Geometry check sheet. Reference: the model listing, model coordinates, mm. A direction names the side the tool comes from. Round coordinates to 2 decimals unless told otherwise and drop trailing zeros. Order: outer loops, then holes, each group sorted by start corner. A loop starts at its lowest first (then second) coordinate and runs counter-clockwise, first axis right, second up. Notation, with made-up numbers: (-18, 18) -> (17, 18) arc R9 cw to (17, 28) -> close; hole circle Ø4 at (19.25, 74). An arc over 180 degrees is marked (long way). Use a Markdown table: item, result. Add a question column.
Item 1: Gauge pin test, flat ends, axial feed: pin 1 Ø5 at (y, z) = (17, -25) entering from -X; pin 2 Ø5 at (x, y) = (-70, 21) entering from -Z; pin 3 Ø6 at (x, y) = (50.5, 13.5) entering from -Z; pin 4 Ø1.2 at (x, z) = (9.28, -18.77) entering from -Y. Record the tip position at first contact, or that the pin passes through.
Item 2: Material ranges on probe 1 along Z at (x, y) = (32, 7.5); probe 2 along Y at (x, z) = (-67, 5); probe 3 along X at (y, z) = (34, -22.5), recorded low to high. Write a range as [from, to].
Item 3: Sectioned sample at D-D, the plane z = 45. Record the cut outline in (x, y), and give its area (3 significant figures).
Item 4: Mould release check, pull along Y, two halves, no side actions. Record for faces 4 (the flat face through (74, 33.55, -26)), 5 (the flat face through (30, 5, 0)), 6 (the flat face through (-15.741, 5, 0)): pulls with the +Y half, pulls with the -Y half, needs draft (parallel to the pull), parting line crosses it, or undercut.
Item 5: Set-up check for faces 1 (the cylindrical face through (-83, 2, 55)), 2 (the flat face through (-74.888, 39, -1)), 3 (the flat face through (59.112, 35, -26)): record each of +Z, -Z, +X, -X, +Y, -Y from which the full face is reachable in a straight line by a thin tool's end or side.
Item 6: Sectioned sample at A-A, the plane x = -85. Record the cut outline in (y, z), and give its area (3 significant figures).
Item 7: Sectioned sample at B-B, the plane z = -36.5. Record the cut outline in (x, y).
Item 8: Sectioned sample at C-C, the plane x = 56. Record the cut outline in (y, z), and give its area (3 significant figures).
from build123d import *

# Parameters (mm, degrees)
SKETCH1_W                           = 180
SKETCH1_H                           = 120
BOSS_EXTRUDE1_DEPTH                 = 10
SKETCH2_W                           = 48.844317462
SKETCH2_H                           = 61.818589288
BOSS_EXTRUDE2_DEPTH                 = 30
SKETCH3_W                           = 27
SKETCH3_H                           = 27
CUT_EXTRUDE1_DEPTH                  = 10
CUT_EXTRUDE5_DEPTH                  = 171.851904114
TAP_DRILL_FOR_M2_5_TAP1_D           = 2.05
TAP_DRILL_FOR_M2_5_TAP1_DEPTH       = 5
TAP_DRILL_FOR_M2_5_TAP1_CSINK_D     = 2.1
TAP_DRILL_FOR_M2_5_TAP1_CSINK_ANGLE = 92
TAP_DRILL_FOR_M2_5_TAP1_TIP         = 0.615882135
CUT_EXTRUDE6_DEPTH                  = 113.249721603
BOSS_EXTRUDE3_DEPTH                 = 49
SKETCH14_W                          = 46
SKETCH14_H                          = 41
CUT_EXTRUDE8_DEPTH                  = 5
TAP_DRILL_FOR_M2_5_TAP2_D           = 2.05
TAP_DRILL_FOR_M2_5_TAP2_DEPTH       = 5
TAP_DRILL_FOR_M2_5_TAP2_CSINK_D     = 2.1
TAP_DRILL_FOR_M2_5_TAP2_CSINK_ANGLE = 92
TAP_DRILL_FOR_M2_5_TAP2_TIP         = 0.615882135
BOSS_EXTRUDE5_DEPTH                 = 115
BOSS_EXTRUDE6_DEPTH                 = 115
SKETCH29_W                          = 30
SKETCH29_H                          = 3.45
BOSS_EXTRUDE10_DEPTH                = 10
SKETCH34_R                          = 2
CUT_EXTRUDE10_DEPTH                 = 5
SKETCH25_R                          = 2
CUT_EXTRUDE11_DEPTH                 = 5
SKETCH36_W                          = 25.507224214
SKETCH36_H                          = 51.818589288
CUT_EXTRUDE12_DEPTH                 = 5
CUT_EXTRUDE14_DEPTH                 = 171.851904114


with BuildPart() as part:
    # Sketch1 → Boss-Extrude1 (new body)
    with BuildSketch(Plane(origin=(0, 0, 0), x_dir=(1, 0, 0), z_dir=(0, 1, 0))):
        Rectangle(SKETCH1_W, SKETCH1_H)
    extrude(amount=BOSS_EXTRUDE1_DEPTH)

    # Sketch2 → Boss-Extrude2 (add)
    with BuildSketch(Plane(origin=(0, 10, 0), x_dir=(1, 0, 0), z_dir=(0, 1, 0))):
        with Locations((-50.466101441, 0)):
            Rectangle(SKETCH2_W, SKETCH2_H)
    extrude(amount=BOSS_EXTRUDE2_DEPTH)

    # Sketch3 → Cut-Extrude1 (cut)
    with BuildSketch(Plane.ZY.offset(74.888260172)):
        with Locations((0, 25)):
            Rectangle(SKETCH3_W, SKETCH3_H)
    extrude(amount=-CUT_EXTRUDE1_DEPTH, mode=Mode.SUBTRACT)

    # Sketch4 → Cut-Extrude5 (cut, through all)
    with BuildSketch(Plane.ZY.offset(64.888260172)):
        with BuildLine():
            Line((-6.024531525, 38.226394973), (5.549516036, 38.226394973))
            ThreePointArc((5.549516036, 38.226394973), (6.551598076, 37.224312933), (5.549516036, 36.222230893))
            Line((5.549516036, 36.222230893), (-6.024531525, 36.222230893))
            ThreePointArc((-6.024531525, 36.222230893), (-7.026613565, 37.224312933), (-6.024531525, 38.226394973))
        make_face()
    extrude(amount=-CUT_EXTRUDE5_DEPTH, mode=Mode.SUBTRACT)

    # Tap Drill for M2.5 Tap1
    with Locations(Plane(origin=(-64.888260172, 36.953397965, -12.070360422), x_dir=(0, 0, -1), z_dir=(-1, 0, 0))):
        with Locations((0, 0), (-24.059553717, -0.049505255), (-23.988973263, 23.863567836), (-0.227588633, 23.863567836)):
            CounterSinkHole(TAP_DRILL_FOR_M2_5_TAP1_D / 2, TAP_DRILL_FOR_M2_5_TAP1_CSINK_D / 2, depth=TAP_DRILL_FOR_M2_5_TAP1_DEPTH, counter_sink_angle=TAP_DRILL_FOR_M2_5_TAP1_CSINK_ANGLE)
            with Locations((0, 0, -(TAP_DRILL_FOR_M2_5_TAP1_DEPTH + TAP_DRILL_FOR_M2_5_TAP1_TIP / 2))):  # 118° drill point
                Cone(0, TAP_DRILL_FOR_M2_5_TAP1_D / 2, TAP_DRILL_FOR_M2_5_TAP1_TIP, mode=Mode.SUBTRACT)

    # Sketch9 → Cut-Extrude6 (cut, through all)
    with BuildSketch(Plane(origin=(0, 10, 0), x_dir=(1, 0, 0), z_dir=(0, 1, 0))):
        with BuildLine():
            Line((-21.846384178, -19.079811509), (-21.846384178, 18.507417164))
            ThreePointArc((-21.846384178, 18.507417164), (-18.793614336, 21.560187005), (-15.740844495, 18.507417164))
            Line((-15.740844495, 18.507417164), (-15.740844495, -19.079811509))
            ThreePointArc((-15.740844495, -19.079811509), (-18.793614336, -22.13258135), (-21.846384178, -19.079811509))
        make_face()
    extrude(amount=-CUT_EXTRUDE6_DEPTH, mode=Mode.SUBTRACT)

    # Sketch10 → Boss-Extrude3 (add)
    with BuildSketch(Plane.ZY.offset(74.888260172)):
        Polygon((30.909294644, 10), (30.909294644, 40), (40.847177304, 10), align=None)
    boss_extrude3 = extrude(amount=-BOSS_EXTRUDE3_DEPTH)

    # Mirror2: Boss-Extrude3 across plane
    add(boss_extrude3.mirror(Plane.XY))

    # Sketch14 → Cut-Extrude8 (cut)
    with BuildSketch(Plane(origin=(0, 10, 0), x_dir=(1, 0, 0), z_dir=(0, 1, 0))):
        with Locations((30.328073167, 0)):
            Rectangle(SKETCH14_W, SKETCH14_H)
    extrude(amount=-CUT_EXTRUDE8_DEPTH, mode=Mode.SUBTRACT)

    # Tap Drill for M2.5 Tap2
    with Locations(Plane(origin=(9.553554548, 5, 18.196456661), x_dir=(0, 0, 1), z_dir=(0, 1, 0))):
        with Locations((0, 0), (-36.962901754, -0.27584255), (-36.549137929, 41.997028299), (0.551685101, 41.997028299)):
            CounterSinkHole(TAP_DRILL_FOR_M2_5_TAP2_D / 2, TAP_DRILL_FOR_M2_5_TAP2_CSINK_D / 2, depth=TAP_DRILL_FOR_M2_5_TAP2_DEPTH, counter_sink_angle=TAP_DRILL_FOR_M2_5_TAP2_CSINK_ANGLE)
            with Locations((0, 0, -(TAP_DRILL_FOR_M2_5_TAP2_DEPTH + TAP_DRILL_FOR_M2_5_TAP2_TIP / 2))):  # 118° drill point
                Cone(0, TAP_DRILL_FOR_M2_5_TAP2_D / 2, TAP_DRILL_FOR_M2_5_TAP2_TIP, mode=Mode.SUBTRACT)

    # Sketch18 → Boss-Extrude5 (add)
    with BuildSketch(Plane(origin=(-25.888260172, 0, 0), x_dir=(0, 0, -1), z_dir=(1, 0, 0))):
        Polygon((40.847177304, 10), (30.909294644, 10), (30.909294644, 40), align=None)
    extrude(amount=BOSS_EXTRUDE5_DEPTH)

    # Sketch19 → Boss-Extrude6 (add)
    with BuildSketch(Plane(origin=(-25.888260172, 0, 0), x_dir=(0, 0, -1), z_dir=(1, 0, 0))):
        Polygon((-30.909294644, 10), (-40.847177304, 10), (-30.909294644, 40), align=None)
    extrude(amount=BOSS_EXTRUDE6_DEPTH)

    # Sketch29 → Boss-Extrude10 (add)
    with BuildSketch(Plane(origin=(0, 0, 30.909294644), x_dir=(-1, 0, 0), z_dir=(0, 0, -1))):
        with Locations((-74.111739828, 35.275)):
            Rectangle(SKETCH29_W, SKETCH29_H)
        with Locations((-74.111739828, 28.825)):
            Rectangle(SKETCH29_W, SKETCH29_H)
    boss_extrude10 = extrude(amount=BOSS_EXTRUDE10_DEPTH)

    # Mirror3: Boss-Extrude10 across plane
    add(boss_extrude10.mirror(Plane.XY))

    # Sketch34 → Cut-Extrude10 (cut)
    with BuildSketch(Plane.XZ):
        with Locations(Location((-85, 55, 0), (0, 0, 270))):
            Circle(SKETCH34_R)
    cut_extrude10 = extrude(amount=-CUT_EXTRUDE10_DEPTH, mode=Mode.SUBTRACT)

    # Sketch25 → Cut-Extrude11 (cut)
    with BuildSketch(Plane.XZ):
        with Locations(Location((85, 55, 0), (0, 0, 270))):
            Circle(SKETCH25_R)
    cut_extrude11 = extrude(amount=-CUT_EXTRUDE11_DEPTH, mode=Mode.SUBTRACT)

    # Mirror4: Cut-Extrude10, Cut-Extrude11 across plane
    add(cut_extrude10.mirror(Plane.XY), mode=Mode.SUBTRACT)
    add(cut_extrude11.mirror(Plane.XY), mode=Mode.SUBTRACT)

    # Sketch36 → Cut-Extrude12 (cut)
    with BuildSketch(Plane(origin=(0, 10, 0), x_dir=(1, 0, 0), z_dir=(0, 1, 0))):
        with Locations((71.865351935, 0)):
            Rectangle(SKETCH36_W, SKETCH36_H)
    extrude(amount=-CUT_EXTRUDE12_DEPTH, mode=Mode.SUBTRACT)

    # Sketch39 → Cut-Extrude14 (cut, through all)
    with BuildSketch(Plane.ZY.offset(64.888260172)):
        with BuildLine():
            Line((-6.024531525, 38.195576912), (5.549516036, 38.195576912))
            ThreePointArc((5.549516036, 38.195576912), (7.522862055, 36.222230893), (5.549516036, 34.248884873))
            Line((5.549516036, 34.248884873), (-6.024531525, 34.248884873))
            ThreePointArc((-6.024531525, 34.248884873), (-7.997877545, 36.222230893), (-6.024531525, 38.195576912))
        make_face()
    extrude(amount=-CUT_EXTRUDE14_DEPTH, mode=Mode.SUBTRACT)


solid = part.part
Found:
| question | item | result |
|---|---|---|
| 1 | pin 1 | stops at x = -74.89 |
| 1 | pin 2 | stops at z = -38.03 |
| 1 | pin 3 | stops at z = -40.68 |
| 1 | pin 4 | passes through |
| 2 | probe 1 | z = [-60, -20.5], [20.5, 60] |
| 2 | probe 2 | y = [0, 11.5], [38.5, 40] |
| 2 | probe 3 | x = [-74.89, -26.04], [59.11, 89.11] |
| 3 | outline | (-90, 0) -> (90, 0) -> (90, 10) -> (-90, 10) -> close |
| 3 | area | 1,800 mm2 |
| 4 | face 4 | undercut |
| 4 | face 5 | pulls with the +Y half |
| 4 | face 6 | needs draft |
| 5 | face 1 | -Y |
| 5 | face 2 | +Z, -Z, -X, +Y |
| 5 | face 3 | +Y |
| 6 | outline | (0, -60) -> (10, -60) -> (10, 60) -> (0, 60) -> (0, 57) -> (5, 57) -> (5, 53) -> (0, 53) -> (0, -53) -> (5, -53) -> (5, -57) -> (0, -57) -> close |
| 6 | area | 1,160 mm2 |
| 7 | outline | (-90, 0) -> (90, 0) -> (90, 10) -> (89.11, 10) -> (89.11, 23.12) -> (-74.89, 23.12) -> (-74.89, 10) -> (-90, 10) -> close |
| 8 | outline | (0, -60) -> (10, -60) -> (10, -40.85) -> (40, -30.91) -> (10, -30.91) -> (10, 30.91) -> (40, 30.91) -> (10, 40.85) -> (10, 60) -> (0, 60) -> close |
| 8 | area | 1,500 mm2 |
